For this review, use the dimensioned drawing (mm, ordinates from the lowest corner) and the shaded views. A direction names the side the tool comes from. Round coordinates to 2 decimals unless told otherwise and drop trailing zeros. Order: outer loops, then holes, each group sorted by start corner. A loop starts at its lowest first (then second) coordinate and runs counter-clockwise, first axis right, second up. Notation, with made-up numbers: (77, -11.5) -> (91, -11.5) arc R18 ccw to (91, 23.5) -> close; hole circle Ø1 at (24, 43.5). An arc over 180 degrees is marked (long way). Answer in a Markdown table with one row per item.
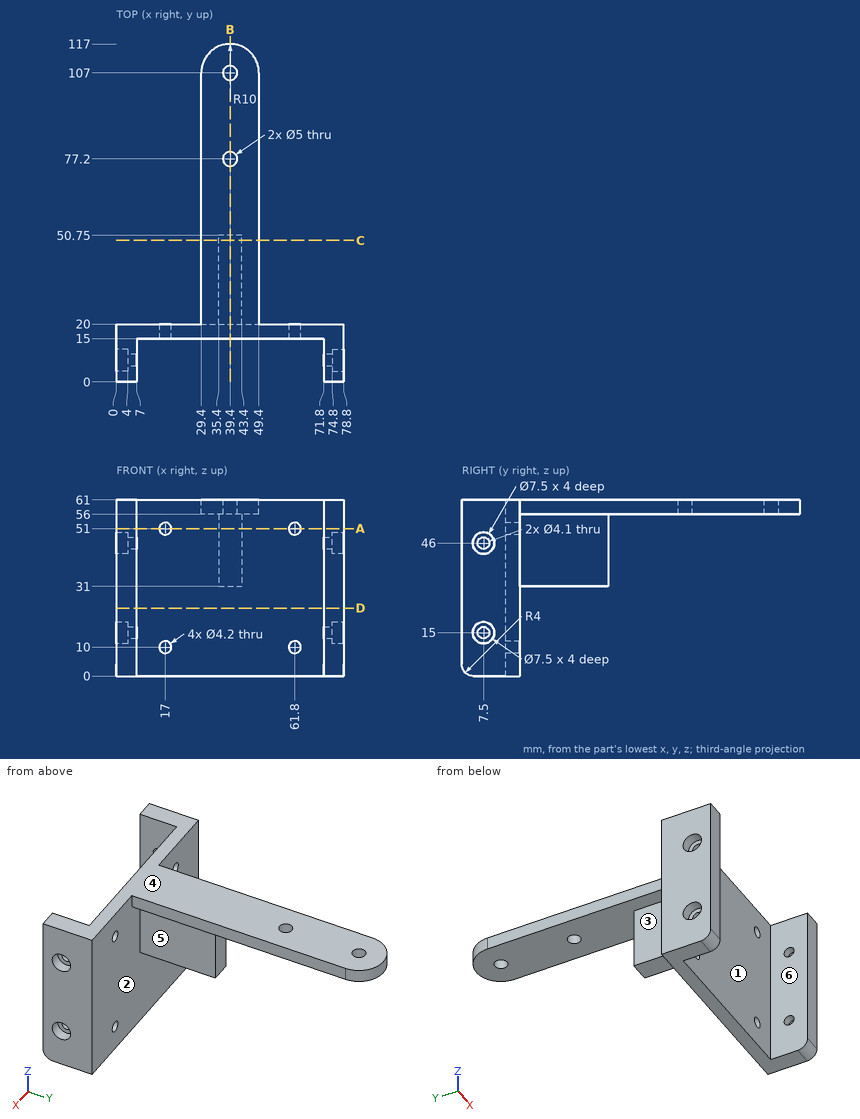
Q1. Take a section at A-A, the plane z = 51. Write out the cut boundary in (x, y).
Answer key:
| item | result |
|---|---|
| outline | (0, 0) -> (7, 0) -> (7, 15) -> (14.9, 15) -> (14.9, 20) -> (0, 20) -> close; (19.1, 15) -> (59.7, 15) -> (59.7, 20) -> (43.4, 20) -> (43.4, 50.75) -> (35.4, 50.75) -> (35.4, 20) -> (19.1, 20) -> close; (63.9, 15) -> (71.8, 15) -> (71.8, 0) -> (78.8, 0) -> (78.8, 20) -> (63.9, 20) -> close |
Q2. Tool access review of the marked faces 4, 5 and 6: name each direction out of +Z, -Z, +X, -X, +Y, -Y from which nothing blocks a thin tool from reaching the whole face with its end or side.
Answer key:
| item | result |
|---|---|
| face 4 | +Z, +X, -X, +Y, -Y |
| face 5 | -Z, +X, +Y |
| face 6 | +Z, -Z, -Y |
Q3. To check wall thickness, follow probe 1 along Z at (x, y) = (17, 17.85); probe 2 along Y at (x, z) = (39, 58); probe 3 along Y at (x, z) = (77.1, 15). State the ranges of each line that lie inside material, in increasing order.
Answer key:
| item | result |
|---|---|
| probe 1 | z = 0 to 7.9, 12.1 to 48.9, 53.1 to 61 |
| probe 2 | y = 15 to 74.73, 79.67 to 104.53, 109.47 to 116.99 |
| probe 3 | y = 0 to 3.75, 11.25 to 20 |
Q4. Take a section at D-D, the plane z = 23.5. Write out the cut boundary in (x, y).
Answer key:
| item | result |
|---|---|
| outline | (0, 0) -> (7, 0) -> (7, 15) -> (71.8, 15) -> (71.8, 0) -> (78.8, 0) -> (78.8, 20) -> (0, 20) -> close |
Q5. Clearance check with flat-ended pins moving along their axes: pin 1 Ø5 at (x, z) = (61.8, 10) entering from +Y; pin 2 Ø10 at (x, z) = (45.5, 45) entering from -Y; pin 3 Ø4 at (y, z) = (9, 46.5) entering from +X. State where each tip first meets the part, or that it passes through.
Answer key:
| item | result |
|---|---|
| pin 1 | stops at y = 20 |
| pin 2 | stops at y = 15 |
| pin 3 | stops at x = 74.8 |
Q6. The part is to be moulded in two halves that separate along X. For the marked faces 1, 2 and 3, say which applies: +X half, -X half, draft (parallel to the pull), parting line (faces both ways), or undercut.
Answer key:
| item | result |
|---|---|
| face 1 | undercut |
| face 2 | draft |
| face 3 | -X half |
Q7. Take a section at B-B, the plane x = 39.4. Write out the cut boundary in (y, z), then the cut area to 3 significant figures.
Answer key:
| item | result |
|---|---|
| outline | (15, 0) -> (20, 0) -> (20, 31) -> (50.75, 31) -> (50.75, 56) -> (74.7, 56) -> (74.7, 61) -> (15, 61) -> close; (79.7, 56) -> (104.5, 56) -> (104.5, 61) -> (79.7, 61) -> close; (109.5, 56) -> (117, 56) -> (117, 61) -> (109.5, 61) -> close |
| area | 1,510 mm^2 |
Q8. Take a section at C-C, the plane y = 49. Write out the cut boundary in (x, z).
Answer key:
| item | result |
|---|---|
| outline | (29.4, 56) -> (35.4, 56) -> (35.4, 31) -> (43.4, 31) -> (43.4, 56) -> (49.4, 56) -> (49.4, 61) -> (29.4, 61) -> close |
